Could you check a few things on this model? Use its own coordinates, in mm. Face numbers are marked on the shaded views. Give positions to 0.01 mm unless a question says otherwise; leave off trailing zeros. Write each loop counter-clockwise with the first axis right and the second up, starting at its lowest first coordinate (ties: lowest second). Pieces come first, ordered by that corner, then holes. Notation, with made-up numbers: M 12,-37 L 32,-37 A27 cw 32,-8 Z; hole C -3,16 d4. An arc over 180 degrees is marked long. Use one line per item in the form item = value.
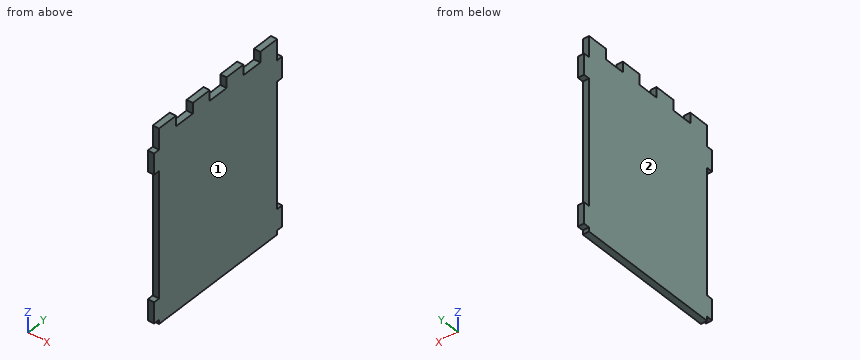
from build123d import *

# Parameters (mm, degrees)
ESBO_O1_W                = 10
ESBO_O1_H                = 3
ESBO_O1_W_2              = 80
ESBO_O1_H_2              = 70
RESSALTO_EXTRUS_O1_DEPTH = 3
ESBO_O2_W                = 2
ESBO_O2_H                = 70
RESSALTO_EXTRUS_O2_DEPTH = 3
ESBO_O3_W                = 5
ESBO_O3_H                = 70
RESSALTO_EXTRUS_O3_DEPTH = 3
ESBO_O4_W                = 5
ESBO_O4_H                = 10
RESSALTO_EXTRUS_O4_DEPTH = 3


with BuildPart() as part:
    # Esboço1 → Ressalto-extrusão1 (new body)
    with BuildSketch(Plane(origin=(0, 0, 0), x_dir=(0, 0, -1), z_dir=(1, 0, 0))):
        with Locations((-35, 36.5)):
            Rectangle(ESBO_O1_W, ESBO_O1_H)
        with Locations((35, 36.5)):
            Rectangle(ESBO_O1_W, ESBO_O1_H)
        with Locations((35, -36.5)):
            Rectangle(ESBO_O1_W, ESBO_O1_H)
        with Locations((-35, -36.5)):
            Rectangle(ESBO_O1_W, ESBO_O1_H)
        Rectangle(ESBO_O1_W_2, ESBO_O1_H_2)
    extrude(amount=RESSALTO_EXTRUS_O1_DEPTH)

    # Esboço2 → Ressalto-extrusão2 (add)
    with BuildSketch(Plane(origin=(3, 0, 0), x_dir=(0, 0, -1), z_dir=(1, 0, 0))):
        with Locations((41, 0)):
            Rectangle(ESBO_O2_W, ESBO_O2_H)
    extrude(amount=-RESSALTO_EXTRUS_O2_DEPTH)

    # Esboço3 → Ressalto-extrusão3 (add)
    with BuildSketch(Plane(origin=(3, 0, 0), x_dir=(0, 0, -1), z_dir=(1, 0, 0))):
        with Locations((-42.5, 0)):
            Rectangle(ESBO_O3_W, ESBO_O3_H)
    extrude(amount=-RESSALTO_EXTRUS_O3_DEPTH)

    # Esboço4 → Ressalto-extrusão4 (add)
    with BuildSketch(Plane(origin=(3, 0, 0), x_dir=(0, 0, -1), z_dir=(1, 0, 0))):
        with Locations((-47.5, 30)):
            Rectangle(ESBO_O4_W, ESBO_O4_H)
        with Locations((-47.5, 10)):
            Rectangle(ESBO_O4_W, ESBO_O4_H)
        with Locations((-47.5, -10)):
            Rectangle(ESBO_O4_W, ESBO_O4_H)
        with Locations((-47.5, -30)):
            Rectangle(ESBO_O4_W, ESBO_O4_H)
    extrude(amount=-RESSALTO_EXTRUS_O4_DEPTH)


solid = part.part
1) For pin 1 Ø1.5 at (x, y) = (2, -37) entering from -Z; pin 2 Ø0.9 at (x, y) = (1.5, 1.5) entering from +Z; pin 3 Ø0.9 at (x, y) = (1, 36.5) entering from +Z, each with a flat end and sliding along its axis, tell me the tip position at first contact or that it passes through.
Checked values:
pin_1 = -40
pin_2 = 45
pin_3 = 40
2) If I drill on L1, parallel to Z at x = 1.8, y = 21; L2, parallel to Y at x = 1.7, z = 24, over which ranges is the centre line in solid material (lowest first)?
Checked values:
L1 = -42 to 45
L2 = -35 to 35
3) I want a section at C-C, the plane z = 17.5. Please give me the cut outline in (x, y).
Checked values:
outline = M 0,-35 L 3,-35 L 3,35 L 0,35 Z
4) Thinking about a two-plate mould opening in X: for the marked faces 1 and 2, which applies, released by +X, released by -X, zero draft, split by the parting line, or undercut?
Checked values:
face_1 = released by +X
face_2 = released by -X
5) I want a section at B-B, the plane y = 4. Please give me the cut outline in (x, z), plus the area to 3 significant figures.
Checked values:
outline = M 0,-42 L 3,-42 L 3,45 L 0,45 Z
area = 261 mm2
